Part model, mm, in its own coordinate system. Face numbers are marked on the shaded views. Round coordinates to 2 decimals unless told otherwise and drop trailing zeros. Loops run counter-clockwise (first coordinate to the right, second up) from the corner with the lowest first, then second, coordinate; pieces in that order, holes last. Notation, with made-up numbers: (11, -31) - (18, -31) arc R11 cw to (18, -24) - close; hole circle Ø10 at (-25.75, 86.25). An arc over 180 degrees is marked (long way). Put each result on its own line as item: value.
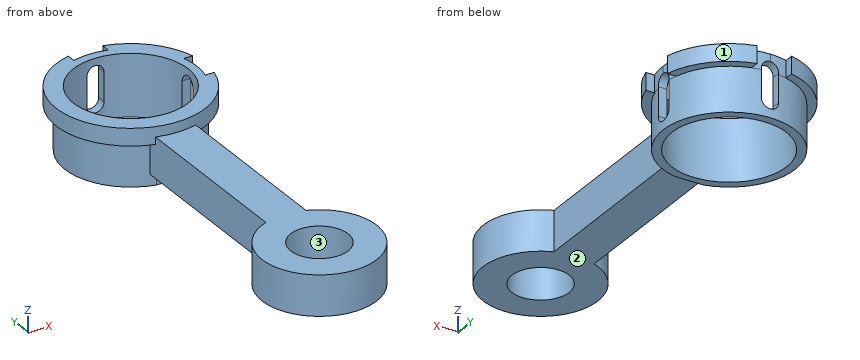
from build123d import *

# Parameters (mm, degrees)
CROQUIS1_R               = 10
SALIENTE_EXTRUIR1_DEPTH  = 3
CROQUIS2_R               = 11.5
CROQUIS2_R_2             = 10
SALIENTE_EXTRUIR3_DEPTH  = 8
SALIENTE_EXTRUIR4_START  = 3
CROQUIS3_R               = 11.5
CROQUIS3_R_2             = 10
SALIENTE_EXTRUIR4_DEPTH  = 3
CORTAR_EXTRUIR1_DEPTH    = 8
SALIENTE_EXTRUIR5_DEPTH  = 8
CORTAR_EXTRUIR2_DEPTH    = 8
CROQUIS11_W              = 0.560243
CROQUIS11_H              = 6
CORTAR_EXTRUIR3_DEPTH    = 8
CROQUIS12_W              = 2.5
CROQUIS12_H              = 0.622045
SALIENTE_EXTRUIR6_DEPTH  = 3
CROQUIS13_W              = 5
CROQUIS13_H              = 50.275028
SALIENTE_EXTRUIR7_DEPTH  = 8
CROQUIS15_W              = 2
CROQUIS15_H              = 50.275028
CORTAR_EXTRUIR4_DEPTH    = 8
SALIENTE_EXTRUIR8_DEPTH  = 7
CROQUIS21_R              = 10
SALIENTE_EXTRUIR9_DEPTH  = 7
CROQUIS22_R              = 5
CORTAR_EXTRUIR5_DEPTH    = 30
CROQUIS23_R              = 10
SALIENTE_EXTRUIR10_DEPTH = 1.25
CORTAR_EXTRUIR6_START    = -1.5
CROQUIS24_R              = 10
CORTAR_EXTRUIR6_DEPTH    = 1.5
SALIENTE_EXTRUIR11_START = -3
CROQUIS25_R              = 13
SALIENTE_EXTRUIR11_DEPTH = 3
CORTAR_EXTRUIR10_DEPTH   = 13
CORTAR_EXTRUIR11_DEPTH   = 13
CORTAR_EXTRUIR14_START   = -10
CROQUIS30_R              = 10
CORTAR_EXTRUIR14_DEPTH   = 10


with BuildPart() as part:
    # Croquis1 → Saliente-Extruir1 (new body)
    with BuildSketch(Plane.XY):
        Circle(CROQUIS1_R)
    extrude(amount=SALIENTE_EXTRUIR1_DEPTH)



with BuildPart() as body_2:
    # Croquis2 → Saliente-Extruir3 (new body)
    with BuildSketch(Plane.XY.offset(3)):
        Circle(CROQUIS2_R)
        Circle(CROQUIS2_R_2, mode=Mode.SUBTRACT)
    extrude(amount=SALIENTE_EXTRUIR3_DEPTH)


with BuildPart() as part_1:
    add(part.part)

    add(body_2.part)  # Saliente-Extruir4 merges body 2
    # Croquis3 → Saliente-Extruir4 (add)
    with BuildSketch(Plane(origin=(0, 0, 3), x_dir=(-1, 0, 0), z_dir=(0, 0, -1)).offset(SALIENTE_EXTRUIR4_START)):
        with Locations(Location((0, 0, 0), (0, 0, 180))):
            Circle(CROQUIS3_R)
        with Locations(Location((0, 0, 0), (0, 0, 180))):
            Circle(CROQUIS3_R_2, mode=Mode.SUBTRACT)
    extrude(amount=-SALIENTE_EXTRUIR4_DEPTH)

    # Croquis4 → Cortar-Extruir1 (cut)
    with BuildSketch(Plane(origin=(0, 11.5, 0), x_dir=(1, 0, 0), z_dir=(0, 1, 0))):
        with BuildLine():
            Line((-1.5, -8), (-1.5, -3))
            ThreePointArc((-1.5, -3), (0, -1.5), (1.5, -3))
            Line((1.5, -3), (1.5, -8))
            ThreePointArc((1.5, -8), (0, -9.5), (-1.5, -8))
        make_face()
    extrude(amount=-CORTAR_EXTRUIR1_DEPTH, mode=Mode.SUBTRACT)


with BuildPart() as body_2_2:
    # Croquis9 → Saliente-Extruir5 (new body)
    with BuildSketch(Plane.XY.offset(11)):
        Polygon((11.5, 0), (11.5, 3), (12.060243, 3), (12.060243, -3), (11.5, -3), align=None)
    extrude(amount=-SALIENTE_EXTRUIR5_DEPTH)


with BuildPart() as cortar_extruir2_tool:
    # Croquis10 → Cortar-Extruir2 (new body)
    with BuildSketch(Plane(origin=(12.060243, 0, 0), x_dir=(0, 0, -1), z_dir=(1, 0, 0))):
        with BuildLine():
            Line((-3, -1.5), (-8, -1.5))
            ThreePointArc((-8, -1.5), (-9.5, 0), (-8, 1.5))
            Line((-8, 1.5), (-3, 1.5))
            ThreePointArc((-3, 1.5), (-1.5, 0), (-3, -1.5))
        make_face()
    extrude(amount=-CORTAR_EXTRUIR2_DEPTH)


with BuildPart() as part_2:
    add(part_1.part)

    # Cortar-Extruir2: cut by cortar_extruir2_tool
    add(cortar_extruir2_tool.part, mode=Mode.SUBTRACT)

    # Croquis12 → Saliente-Extruir6 (add)
    with BuildSketch(Plane.XY.offset(3)):
        with Locations((-1.25, -11.188978)):
            Rectangle(CROQUIS12_W, CROQUIS12_H)
        with Locations((1.25, -11.188978)):
            Rectangle(CROQUIS12_W, CROQUIS12_H)
        Polygon((2.5, -11.5), (2.5, -61.5), (-2.5, -61.5), (-2.5, -11.5), (0, -11.5), align=None)
    extrude(amount=-SALIENTE_EXTRUIR6_DEPTH)

    # Croquis13 → Saliente-Extruir7 (add)
    with BuildSketch(Plane.XY.offset(3)):
        with Locations((0, -36.362486)):
            Rectangle(CROQUIS13_W, CROQUIS13_H)
    extrude(amount=SALIENTE_EXTRUIR7_DEPTH)

    # Croquis15 → Cortar-Extruir4 (cut)
    with BuildSketch(Plane(origin=(2.5, 0, 0), x_dir=(0, 0, -1), z_dir=(1, 0, 0))):
        with Locations((-10, -36.362486)):
            Rectangle(CROQUIS15_W, CROQUIS15_H)
        with Locations((-1, -36.362486)):
            Rectangle(CROQUIS15_W, CROQUIS15_H)
    extrude(amount=-CORTAR_EXTRUIR4_DEPTH, mode=Mode.SUBTRACT)

    # Croquis16 → Saliente-Extruir8 (add)
    with BuildSketch(Plane.XY.offset(9)):
        Polygon((-2.5, -61.5), (-3.5, -61.5), (-3.5, -10.232956), (3.5, -10.232956), (3.5, -61.5), (2.5, -61.5), align=None)
    extrude(amount=-SALIENTE_EXTRUIR8_DEPTH)

    # Croquis21 → Saliente-Extruir9 (add)
    with BuildSketch(Plane(origin=(0, 0, 2), x_dir=(-1, 0, 0), z_dir=(0, 0, -1))):
        with Locations((0, -52.724972)):
            Circle(CROQUIS21_R)
    extrude(amount=-SALIENTE_EXTRUIR9_DEPTH)

    # Croquis22 → Cortar-Extruir5 (cut)
    with BuildSketch(Plane(origin=(0, 0, 2), x_dir=(-1, 0, 0), z_dir=(0, 0, -1))):
        with Locations((0, -52.724972)):
            Circle(CROQUIS22_R)
    extrude(amount=-CORTAR_EXTRUIR5_DEPTH, mode=Mode.SUBTRACT)

    # Croquis23 → Saliente-Extruir10 (add)
    with BuildSketch(Plane.XY.offset(11)):
        with BuildLine():
            Line((-2.5, -11.224972), (2.5, -11.224972))
            ThreePointArc((2.5, -11.224972), (0, 11.5), (-2.5, -11.224972))
        make_face()
        with Locations(Location((0, 0, 0), (0, 0, 98.626927))):
            Circle(CROQUIS23_R, mode=Mode.SUBTRACT)
    extrude(amount=SALIENTE_EXTRUIR10_DEPTH)

    # Croquis24 → Cortar-Extruir6 (cut)
    with BuildSketch(Plane.XY.offset(12.25).offset(CORTAR_EXTRUIR6_START)):
        with BuildLine():
            Line((-2.5, -11.224972), (2.5, -11.224972))
            ThreePointArc((2.5, -11.224972), (0, 11.5), (-2.5, -11.224972))
        make_face()
        with Locations(Location((0, 0, 0), (0, 0, 98.626927))):
            Circle(CROQUIS24_R, mode=Mode.SUBTRACT)
    extrude(amount=CORTAR_EXTRUIR6_DEPTH, mode=Mode.SUBTRACT)

    # Croquis25 → Saliente-Extruir11 (add)
    with BuildSketch(Plane.XY.offset(10.75).offset(SALIENTE_EXTRUIR11_START)):
        Circle(CROQUIS25_R)
        with BuildLine():
            ThreePointArc((2.5, -11.224972), (0, 11.5), (-2.5, -11.224972))
            Line((-2.5, -11.224972), (2.5, -11.224972))
        make_face(mode=Mode.SUBTRACT)
    extrude(amount=SALIENTE_EXTRUIR11_DEPTH)

    # Croquis27 → Cortar-Extruir10 (cut)
    with BuildSketch(Plane(origin=(0, 0, 0), x_dir=(-1, 0, 0), z_dir=(0, 0, -1))):
        with BuildLine():
            ThreePointArc((-3, 11.101802), (-1.513156, 11.400016), (0, 11.5))
            Line((0, 11.5), (-3, 11.5))
            Line((-3, 11.5), (-3, 11.369881))
            Line((-3, 11.369881), (-3, 11.101802))
        make_face()
        with BuildLine():
            Line((3, 11.369881), (3, 11.5))
            Line((3, 11.5), (0, 11.5))
            ThreePointArc((0, 11.5), (1.513156, 11.400016), (3, 11.101802))
            Line((3, 11.101802), (3, 11.369881))
        make_face()
        Polygon((0, 11.5), (3, 11.5), (3, 12.649111), (3, 13.586373), (-0.001501, 13.586373), (-3, 13.586373), (-3, 11.5), align=None)
    extrude(amount=-CORTAR_EXTRUIR10_DEPTH, mode=Mode.SUBTRACT)

    # Croquis28 → Cortar-Extruir11 (cut)
    with BuildSketch(Plane(origin=(0, 0, 0), x_dir=(-1, 0, 0), z_dir=(0, 0, -1))):
        Polygon((-13.802598, 3), (-11.5, 3), (-11.5, 0), (-11.5, -3), (-13.802598, -3), align=None)
        with BuildLine():
            Line((-11.5, 3), (-11.5, 0))
            ThreePointArc((-11.5, 0), (-11.400016, 1.513156), (-11.101802, 3))
            Line((-11.101802, 3), (-11.5, 3))
        make_face()
        with BuildLine():
            ThreePointArc((-11.101802, -3), (-11.400016, -1.513156), (-11.5, 0))
            Line((-11.5, 0), (-11.5, -3))
            Line((-11.5, -3), (-11.101802, -3))
        make_face()
    extrude(amount=-CORTAR_EXTRUIR11_DEPTH, mode=Mode.SUBTRACT)

    # Croquis30 → Cortar-Extruir14 (cut)
    with BuildSketch(Plane.XY.offset(3).offset(CORTAR_EXTRUIR14_START)):
        Circle(CROQUIS30_R)
    extrude(amount=CORTAR_EXTRUIR14_DEPTH, mode=Mode.SUBTRACT)


with BuildPart() as body_2_2_1:
    add(body_2_2.part)

    # Cortar-Extruir2: cut by cortar_extruir2_tool
    add(cortar_extruir2_tool.part, mode=Mode.SUBTRACT)

    # Croquis11 → Cortar-Extruir3 (cut)
    with BuildSketch(Plane.XY.offset(11)):
        with Locations((11.780121, 0)):
            Rectangle(CROQUIS11_W, CROQUIS11_H)
    extrude(amount=-CORTAR_EXTRUIR3_DEPTH, mode=Mode.SUBTRACT)


solid = part_2.part
1. Pin check, flat tips, straight feed: P1, Ø0.8, axis at x = 11.5, z = 9.5, coming from the +Y side; P2, Ø10.5, axis at x = 7.5, y = 7.5, coming from the -Z side; P3, Ø0.8, axis at y = 12, z = 9, coming from the -X side; P4, Ø3, axis at y = -18, z = 7, coming from the +X side. Stop position of each tip, or through.
A:
P1: stops at y = 6.77
P2: stops at z = 0
P3: stops at x = -5.87
P4: stops at x = 3.5
2. Band-saw the part on A-A (z = 5.75). List the corners of the cut face in (x, y).
A:
outline: (-3.5, -43.36) arc R10 ccw (long way) to (3.5, -43.36) - (3.5, -10.95) arc R11.5 ccw to (11.4, -1.5) - (9.89, -1.5) arc R10 cw (long way) to (-1.5, 9.89) - (-1.5, 11.4) arc R11.5 ccw to (-3.5, -10.95) - close; (1.5, 9.89) arc R10 cw to (9.89, 1.5) - (11.4, 1.5) arc R11.5 ccw to (1.5, 11.4) - close; hole circle Ø10 at (0, -52.72)
3. Probe line 1 along Y through (x, z) = (0, 7); line 2 along Y through (x, z) = (6, 5); line 3 along Y through (x, z) = (-6.25, 2.25). List the from-to ranges inside material, lowest first. Write a range as [from, to].
A:
line 1: y = [-62.72, -57.72], [-47.72, -10]
line 2: y = [-60.72, -44.72], [-9.81, -8], [8, 9.81]
line 3: y = [-60.53, -44.92], [-9.65, -7.81], [7.81, 9.65]
4. Band-saw the part on B-B (y = -18.5). List the corners of the cut face in (x, z).
A:
outline: (-3.5, 2) - (3.5, 2) - (3.5, 9) - (-3.5, 9) - close
5. Two-plate mould, pull along Y, no slides. Class the marked faces 1, 2 and 3: pulls with the +Y half, pulls with the -Y half, needs draft (parallel to the pull), parting line crosses it, or undercut.
A:
face 1: pulls with the +Y half
face 2: needs draft
face 3: undercut
